from build123d import *

# Parameters (mm, degrees)
CROQUIS1_R              = 20
SALIENTE_EXTRUIR1_DEPTH = 3
CROQUIS2_R              = 20
CROQUIS2_R_2            = 7
SALIENTE_EXTRUIR2_DEPTH = 50
CROQUIS6_W              = 2
CROQUIS6_H              = 12
CORTAR_EXTRUIR1_DEPTH   = 32


with BuildPart() as part:
    # Croquis1 → Saliente-Extruir1 (new body)
    with BuildSketch(Plane.XY):
        with Locations((-44.21130789, 7.297319347)):
            Circle(CROQUIS1_R)
    extrude(amount=SALIENTE_EXTRUIR1_DEPTH)

    # Croquis2 → Saliente-Extruir2 (add)
    with BuildSketch(Plane.XY.offset(3)):
        with Locations((-44.21130789, 7.297319347)):
            Circle(CROQUIS2_R)
        with Locations((-44.21130789, 17.297319347)):
            Circle(CROQUIS2_R_2, mode=Mode.SUBTRACT)
        with Locations((-34.21130789, 7.297319347)):
            Circle(CROQUIS2_R_2, mode=Mode.SUBTRACT)
        with Locations((-44.21130789, -2.702680653)):
            Circle(CROQUIS2_R_2, mode=Mode.SUBTRACT)
        with Locations((-54.21130789, 7.297319347)):
            Circle(CROQUIS2_R_2, mode=Mode.SUBTRACT)
    extrude(amount=SALIENTE_EXTRUIR2_DEPTH)

    # Croquis4 → Revolución1 (revolve)
    with BuildSketch(Plane(origin=(0, 7.297319347, 0), x_dir=(1, 0, 0), z_dir=(0, 1, 0))):
        with BuildLine():
            Line((-48.21130789, 0), (-64.21130789, 0))
            ThreePointArc((-64.21130789, 0), (-53.677160121, 18.986340893), (-48.21130789, 40))
            Line((-48.21130789, 40), (-48.21130789, 0))
        make_face()
    revolve(axis=Axis((-44.21130789, 7.297319347, 0), (0, 0, -1)))

    # Croquis6 → Cortar-Extruir1 (cut)
    with BuildSketch(Plane(origin=(-11.912562698, 11.676862537, 0), x_dir=(0, 0, -1), z_dir=(0.714136384, -0.700006589, 0))):
        with Locations((-4, -17.736925603)):
            Rectangle(CROQUIS6_W, CROQUIS6_H)
        with Locations((-4, -33.736925603)):
            Rectangle(CROQUIS6_W, CROQUIS6_H)
    extrude(amount=-CORTAR_EXTRUIR1_DEPTH, mode=Mode.SUBTRACT)


solid = part.part
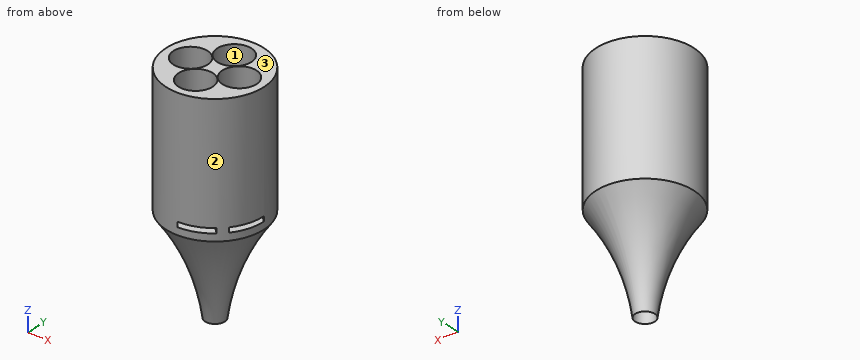
Geometry check sheet. Reference: the model listing, model coordinates, mm. Face numbers are marked on the shaded views. Coordinates: 2 decimals unless noted, no trailing zeros. Order: outer loops, then holes, each group sorted by start corner. A loop starts at its lowest first (then second) coordinate and runs counter-clockwise, first axis right, second up. Notation, with made-up numbers: (-1.75, 49.5) - (30.25, 49.5) arc R12 ccw to (30.25, 62.5) - close; hole circle Ø7 at (61.5, 69). An arc over 180 degrees is marked (long way). One line per item, written item: value.
(1) Release check for a two-part mould opening along Y. For the marked faces 1, 2 and 3 record: +Y half, -Y half, draft (parallel to the pull), parting line (faces both ways), or undercut.
Data:
face 1: undercut
face 2: parting line
face 3: draft
(2) Sectioned sample at B-B (z = -7.5). Enter the section's corners in (x, y), and give its area (3 significant figures).
Data:
outline: circle Ø30.16 at (-44.21, 7.3); hole circle Ø8 at (-44.21, 7.3)
area: 664 mm^2
(3) Sectioned sample at A-A (z = 18). Enter the section's corners in (x, y).
Data:
outline: circle Ø40 at (-44.21, 7.3); hole circle Ø14 at (-54.21, 7.3); hole circle Ø14 at (-44.21, -2.7); hole circle Ø14 at (-44.21, 17.3); hole circle Ø14 at (-34.21, 7.3)
(4) Depth check by flat-ended pin: pin 1 Ø8 at (x, y) = (-29, 5) entering from -Z; pin 2 Ø0.8 at (x, y) = (-42, 24.5) entering from -Z; pin 3 Ø10 at (x, z) = (-30.5, -7) entering from +Y. Enter the tip coordinate at first touch or a pass-through.
Data:
pin 1: stops at z = -14.55
pin 2: stops at z = -4.45
pin 3: stops at y = 21.65
(5) Thickness scan on probe 1 along Y at (x, z) = (-48, 48.5); probe 2 along Y at (x, z) = (-46, 39.5); probe 3 along Y at (x, z) = (-50, 28). Record the ranges inside material, lowest first. Write a range as from..to.
Data:
probe 1: y = -12.34..-8.59, 3.18..4.07, 10.53..11.41, 23.18..26.94
probe 2: y = -12.62..-9.47, 4.06..10.53, 24.06..27.22
probe 3: y = -11.85..-6.64, 1.23..1.71, 12.89..13.36, 21.23..26.44
(6) Sectioned sample at C-C (z = -29). Enter the section's corners in (x, y), and give its area (3 significant figures).
Data:
outline: circle Ø12.31 at (-44.21, 7.3); hole circle Ø8 at (-44.21, 7.3)
area: 68.7 mm^2
